Build history of the part. All positions in model axes, mm. Round coordinates to 2 decimals unless told otherwise and drop trailing zeros. Loops run counter-clockwise (first coordinate to the right, second up) from the corner with the lowest first, then second, coordinate; pieces in that order, holes last. Notation, with made-up numbers: (56, -11.5) - (67, -11.5) arc R19 ccw to (67, 5.5) - close; hole circle Ø3 at (0, -36.75). An arc over 180 degrees is marked (long way). Put each result on its own line as item: value. Start each with the question number.
from build123d import *

# Parameters (mm, degrees)
SKETCH2_W           = 133.35
SKETCH2_H           = 160.866666666
SKETCH2_W_2         = 93.133333333
SKETCH2_H_2         = 135.466666666
SKETCH2_W_3         = 8.466666667
BOSS_EXTRUDE1_DEPTH = 12.7
CUT_EXTRUDE1_DEPTH  = 6.35
CHAMFER4_SIZE       = 3.81
CHAMFER1_SIZE       = 0.635
CHAMFER2_SIZE       = 3.175
SKETCH4_W           = 8.89
SKETCH4_H           = 11.43
CUT_EXTRUDE2_DEPTH  = 10.16
SKETCH5_W           = 8.89
SKETCH5_H           = 11.43
CUT_EXTRUDE3_DEPTH  = 10.16
SKETCH6_W           = 12.7
SKETCH6_H           = 124.46
BOSS_EXTRUDE2_DEPTH = 2.286
CHAMFER5_SIZE       = 2.286


with BuildPart() as part:
    # Sketch2 → Boss-Extrude1 (new body)
    with BuildSketch(Plane(origin=(0, 0, 0), x_dir=(1, 0, 0), z_dir=(0, 1, 0))):
        Rectangle(SKETCH2_W, SKETCH2_H)
        with Locations((-7.408333333, 0)):
            Rectangle(SKETCH2_W_2, SKETCH2_H_2, mode=Mode.SUBTRACT)
        with Locations((49.741666667, 0)):
            Rectangle(SKETCH2_W_3, SKETCH2_H_2, mode=Mode.SUBTRACT)
    extrude(amount=BOSS_EXTRUDE1_DEPTH)

    # Sketch3 → Cut-Extrude1 (cut)
    with BuildSketch(Plane.XZ):
        Polygon((-57.15, 76.2), (-60.325, 73.025), (-63.5, 76.2), (-60.325, 79.375), align=None)
        Polygon((57.15, 76.2), (53.975, 73.025), (50.8, 76.2), (53.975, 79.375), align=None)
        Polygon((63.5, -76.2), (60.325, -79.375), (57.15, -76.2), (60.325, -73.025), align=None)
        Polygon((-57.15, -76.2), (-60.325, -79.375), (-63.5, -76.2), (-60.325, -73.025), align=None)
    extrude(amount=-CUT_EXTRUDE1_DEPTH, mode=Mode.SUBTRACT)

    # Chamfer4
    chamfer4_edges = [part.edges().sort_by_distance(p)[0] for p in [
        (0, 12.7, -80.433333333),
        (0, 12.7, 80.433333333),
    ]]
    chamfer(chamfer4_edges, length=CHAMFER4_SIZE)

    # Chamfer1
    chamfer1_edges = [part.edges().sort_by_distance(p)[0] for p in [
        (-58.7375, 6.35, -74.6125),
        (-58.7375, 6.35, -77.7875),
        (-61.9125, 6.35, -77.7875),
        (-61.9125, 6.35, -74.6125),
        (-58.7375, 0, -74.6125),
        (-61.9125, 0, -74.6125),
        (-61.9125, 0, -77.7875),
        (-58.7375, 0, -77.7875),
        (61.9125, 6.35, -74.6125),
        (61.9125, 6.35, -77.7875),
        (58.7375, 6.35, -77.7875),
        (58.7375, 6.35, -74.6125),
        (61.9125, 0, -74.6125),
        (58.7375, 0, -74.6125),
        (58.7375, 0, -77.7875),
        (61.9125, 0, -77.7875),
        (55.5625, 6.35, 77.7875),
        (55.5625, 6.35, 74.6125),
        (52.3875, 6.35, 74.6125),
        (52.3875, 6.35, 77.7875),
        (55.5625, 0, 77.7875),
        (52.3875, 0, 77.7875),
        (52.3875, 0, 74.6125),
        (55.5625, 0, 74.6125),
        (-58.7375, 6.35, 77.7875),
        (-58.7375, 6.35, 74.6125),
        (-61.9125, 6.35, 74.6125),
        (-61.9125, 6.35, 77.7875),
        (-58.7375, 0, 77.7875),
        (-61.9125, 0, 77.7875),
        (-61.9125, 0, 74.6125),
        (-58.7375, 0, 74.6125),
    ]]
    chamfer(chamfer1_edges, length=CHAMFER1_SIZE)

    # Chamfer2
    chamfer2_edges = [part.edges().sort_by_distance(p)[0] for p in [
        (53.975, 0, 0),
        (49.741666667, 0, -67.733333333),
        (49.741666667, 0, 67.733333333),
        (-7.408333333, 0, -67.733333333),
        (-53.975, 0, 0),
        (-7.408333333, 0, 67.733333333),
    ]]
    chamfer(chamfer2_edges, length=CHAMFER2_SIZE)

    # Sketch4 → Cut-Extrude2 (cut)
    with BuildSketch(Plane.XY.offset(80.433333333)):
        with Locations((38.0365, 6.985)):
            Rectangle(SKETCH4_W, SKETCH4_H)
    extrude(amount=-CUT_EXTRUDE2_DEPTH, mode=Mode.SUBTRACT)

    # Sketch5 → Cut-Extrude3 (cut)
    with BuildSketch(Plane(origin=(0, 0, -80.433333333), x_dir=(-1, 0, 0), z_dir=(0, 0, -1))):
        with Locations((-38.0365, 6.985)):
            Rectangle(SKETCH5_W, SKETCH5_H)
    extrude(amount=-CUT_EXTRUDE3_DEPTH, mode=Mode.SUBTRACT)

    # Sketch6 → Boss-Extrude2 (add)
    with BuildSketch(Plane(origin=(0, 12.7, 0), x_dir=(1, 0, 0), z_dir=(0, 1, 0))):
        with Locations((-60.325, 0)):
            Rectangle(SKETCH6_W, SKETCH6_H)
    extrude(amount=BOSS_EXTRUDE2_DEPTH)

    # Chamfer5
    chamfer5_edges = [part.edges().sort_by_distance(p)[0] for p in [
        (-60.325, 14.986, -62.23),
        (-60.325, 14.986, 62.23),
    ]]
    chamfer(chamfer5_edges, length=CHAMFER5_SIZE - 0.0001)  # a hair under: the kernel refuses the full size


solid = part.part
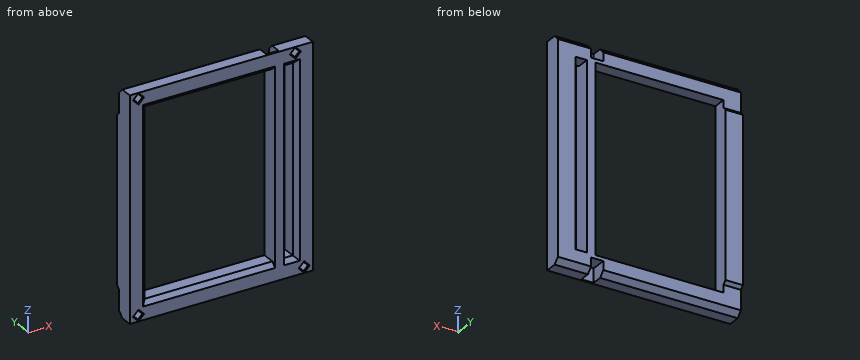
Item 1: Slice it at A-A (z = -5.5). Give the cut face in (x, y) (3 decimals), plus the area to 3 significant figures.
Item 2: Slice it at C-C (y = 11). Give the cut face in (x, z) (1 decimal), plus the area to 3 significant figures.
Item 3: Drill centre lines: probe 1 along X at (y, z) = (4.5, -10) (3 decimals); probe 2 along Z at (x, y) = (-29.5, 6.5); probe 3 along X at (y, z) = (2.5, -17.5) (3 decimals). Where is each one in solid material? Low to high. Write a range as [from, to].
Item 4: Slice it at B-B (x = 25). Give the cut face in (y, z) (3 decimals), plus the area to 3 significant figures.
Item 5: Drop flat-ended pins along their axis: pin 1 Ø2.5 at (x, z) = (36.5, -76) entering from +Y; pin 2 Ø3.5 at (x, z) = (60.5, -76.5) entering from -Y; pin 3 Ø7 at (x, y) = (49.5, 10) entering from -Z; pin 4 Ø2 at (x, z) = (45, 54.5) entering from +Y. Give the stop position or say it passes through.
Computed values:
1. outline: (-66.675, 0) - (-57.15, 0) - (-53.975, 3.175) - (-53.975, 14.986) - (-66.675, 14.986) - close; (39.158, 0) - (45.508, 0) - (45.508, 12.7) - (39.158, 12.7) - close; (53.975, 3.175) - (57.15, 0) - (66.675, 0) - (66.675, 12.7) - (53.975, 12.7) - close
1. area: 422 mm^2
2. outline: (-66.7, -78.3) - (33.6, -78.3) - (33.6, -70.3) - (42.5, -70.3) - (42.5, -78.3) - (66.7, -78.3) - (66.7, 78.3) - (42.5, 78.3) - (42.5, 70.3) - (33.6, 70.3) - (33.6, 78.3) - (-66.7, 78.3) - close; hole (-54, -67.7) - (39.2, -67.7) - (39.2, 67.7) - (-54, 67.7) - close; hole (45.5, -67.7) - (54, -67.7) - (54, 67.7) - (45.5, 67.7) - close
2. area: 6,980 mm^2
3. probe 1: x = [-66.675, -53.975], [39.158, 45.508], [53.975, 66.675]
3. probe 2: z = [-80.43, -67.73], [67.73, 80.43]
3. probe 3: x = [-66.675, -54.65], [39.158, 45.508], [54.65, 66.675]
4. outline: (0, -80.433) - (8.89, -80.433) - (12.7, -76.623) - (12.7, -67.733) - (3.175, -67.733) - (0, -70.908) - close; (0, 70.908) - (3.175, 67.733) - (12.7, 67.733) - (12.7, 76.623) - (8.89, 80.433) - (0, 80.433) - close
4. area: 298 mm^2
5. pin 1: stops at y = 1.27
5. pin 2: stops at y = 5.87
5. pin 3: stops at z = -80.43
5. pin 4: stops at y = 12.7
